Input: part model. Units: mm. Frame: model coordinates. A direction names the side the tool comes from. Coordinates: 2 decimals unless noted, no trailing zeros. Order: outer loops, then holes, each group sorted by start corner. A loop starts at its lowest first (then second) coordinate and runs counter-clockwise, first axis right, second up.
from build123d import *

# Parameters (mm, degrees)
F0_W     = 76.2
F0_H     = 101.6
F1_DEPTH = 12.7
F2_W     = 63.9262623101
F2_H     = 12.7
F3_DEPTH = 50.8
F4_DEPTH = 35.56
F5_R     = 19.05
F6_DEPTH = 38.101
F7_R     = 38.09999


# Not quite as in the source:
# - a fillet or chamfer is up to 0.001 mm smaller than in the source, because OpenCascade refuses the exact size


with BuildPart() as f1:
    # F0 (on Top) → F1 (new body)
    with BuildSketch(Plane.XY):
        Rectangle(F0_W, F0_H)
    extrude(amount=F1_DEPTH)

    # F2 (on Front) → F3 (join)
    with BuildSketch(Plane.XZ):
        Polygon((-25.8262623101, 25.4), (-38.1, 25.4), (-38.1, 12.7), (38.1, 12.7), (38.1, 25.4), align=None)
        with Locations((6.1368688449, 31.75)):
            Rectangle(F2_W, F2_H)
    extrude(amount=-F3_DEPTH)

    # F4 (cut): a face of the model
    f4_faces = [f1.faces().sort_by_distance(p)[0] for p in [
        (2.7996685352, 0, 24.8437999484),
    ]]
    extrude(f4_faces, amount=-F4_DEPTH, mode=Mode.SUBTRACT)

    # F5 (on Top) → F6 (cut, through all)
    with BuildSketch(Plane.XY):
        with Locations((0, -19.05)):
            Circle(F5_R)
    extrude(amount=F6_DEPTH, mode=Mode.SUBTRACT)

    # F7 (radius 38.1 in the source; OpenCascade refuses exactly that, so slightly less here)
    f7_edges = [f1.edges().sort_by_distance(p)[0] for p in [
        (-38.1, -50.8, 6.35),
        (38.1, -50.8, 6.35),
    ]]
    fillet(f7_edges, radius=F7_R)


solid = f1.part
Item 1: Cut plane D-D on y = -28. Return loops of the section in (x, z).
Response values:
outline: (-34.89, 0) - (-16.82, 0) - (-16.82, 12.7) - (-34.89, 12.7) - close; (16.82, 0) - (34.89, 0) - (34.89, 12.7) - (16.82, 12.7) - close
Item 2: Pin query (flat end, axial travel): pin 1 Ø1 at (x, z) = (10.5, 20.5) entering from -Y; pin 2 Ø13.5 at (x, y) = (-32.5, 44.5) entering from +Z; pin 3 Ø10 at (y, z) = (8.5, 19) entering from +X; pin 4 Ø10 at (y, z) = (46.5, 33.5) entering from -X. Return the tip coordinate at first contact, or that it passes through.
Response values:
pin 1: stops at y = 35.56
pin 2: stops at z = 38.1
pin 3: passes through
pin 4: stops at x = -25.83
Item 3: Ray query, probe 1 along Y at (x, z) = (0, 8.75); probe 2 along Z at (x, y) = (7.5, 10.5); probe 3 along X at (y, z) = (-19.05, 5.25). Return the intervals inside material, ascending.
Response values:
probe 1: y = -50.8 to -38.1, 0 to 50.8
probe 2: z = 0 to 12.7
probe 3: x = -37.57 to -19.05, 19.05 to 37.57
Item 4: Draft query along X for faces 1 (the face through (-4.13, -37.647, 6.261)), 2 (the face through (-25.826, 43, 32)), 3 (the face through (-1, 1, 12.7)), 4 (the face through (38.1, 26, 10)). Return one class per face: pulls with the +X half, pulls with the -X half, needs draft (parallel to the pull), parting line crosses it, or undercut.
Response values:
face 1: undercut
face 2: pulls with the -X half
face 3: needs draft
face 4: pulls with the +X half
Item 5: Cut plane C-C on z = 17. Return loops of the section in (x, y).
Response values:
outline: (-38.1, 35.56) - (38.1, 35.56) - (38.1, 50.8) - (-38.1, 50.8) - close
Item 6: Cut plane A-A on y = -11.5. Return loops of the section in (x, z), then the cut area to 3 significant figures.
Response values:
outline: (-38.1, 0) - (-17.49, 0) - (-17.49, 12.7) - (-38.1, 12.7) - close; (17.49, 0) - (38.1, 0) - (38.1, 12.7) - (17.49, 12.7) - close
area: 523 mm2
Item 7: Access query for faces 5 (the face through (-32, 43, 25.4)), 6 (the face through (26.64, -39.94, 6.44)), 7 (the face through (-1, 35.56, 26)). Directions: +Z, -Z, +X, -X, +Y, -Y. A direction counts if a zero-diameter tool reaches every point of the face in a straight line with its end or side. Return the directions, or none.
Response values:
face 5: +Z, -X, +Y, -Y
face 6: +Z, -Z, +X, -Y
face 7: +Z, +X, -X, -Y
